Here's how the part is built. I have some questions about the finished solid (model axes, mm). A direction names the side the tool comes from. Round coordinates to 2 decimals unless told otherwise and drop trailing zeros. Loops run counter-clockwise (first coordinate to the right, second up) from the corner with the lowest first, then second, coordinate; pieces in that order, holes last. Notation, with made-up numbers: M 82,88.25 L 129,88.25 A25 ccw 129,101.25 Z; hole C 48.25,11 d11. An arc over 180 degrees is marked long. Put each result on its own line as item: value. Start each with the question number.
```python
from build123d import *

# Parameters (mm, degrees)
SKETCH_1_R          = 2
SKETCH_1_R_2        = 1
EXTRUDE_1_DEPTH     = 29
SKETCH_2_R          = 3
SKETCH_2_R_2        = 2
EXTRUDE_2_DEPTH     = 2.5
EXTRUDE_START       = 26.5
SKETCH_3_R          = 3
SKETCH_3_R_2        = 2
EXTRUDE_3_DEPTH     = 2.5
SKETCH_4_R          = 1.6
CUT_EXTRUDE_1_DEPTH = 1.5
CUT_EXTRUDE_START   = 29
CUT_EXTRUDE_2_DEPTH = 1.6
CUT_EXTRUDE_START_2 = 18.5
SKETCH_7_R          = 3
CUT_EXTRUDE_3_DEPTH = 10.5
CUT_EXTRUDE_START_3 = 10.5
CUT_EXTRUDE_5_DEPTH = 8


with BuildPart() as part:
    # 草图1 → 凸台-拉伸1 (new body)
    with BuildSketch(Plane(origin=(0, 0, 0), x_dir=(1, 0, 0), z_dir=(0, 1, 0))):
        with Locations(Location((0, 0, 0), (0, 0, 90))):
            Circle(SKETCH_1_R)
        with Locations(Location((0, 0, 0), (0, 0, 90))):
            Circle(SKETCH_1_R_2, mode=Mode.SUBTRACT)
    extrude(amount=EXTRUDE_1_DEPTH)

    # 草图2 → 凸台-拉伸2 (add)
    with BuildSketch(Plane(origin=(0, 0, 0), x_dir=(1, 0, 0), z_dir=(0, 1, 0))):
        with Locations(Location((0, 0, 0), (0, 0, 270))):
            Circle(SKETCH_2_R)
        with Locations(Location((0, 0, 0), (0, 0, 90))):
            Circle(SKETCH_2_R_2, mode=Mode.SUBTRACT)
    extrude(amount=EXTRUDE_2_DEPTH)

    # 草图3 → 凸台-拉伸3 (add)
    with BuildSketch(Plane(origin=(0, 0, 0), x_dir=(1, 0, 0), z_dir=(0, 1, 0)).offset(EXTRUDE_START)):
        with Locations(Location((0, 0, 0), (0, 0, 270))):
            Circle(SKETCH_3_R)
        with Locations(Location((0, 0, 0), (0, 0, 90))):
            Circle(SKETCH_3_R_2, mode=Mode.SUBTRACT)
    extrude(amount=EXTRUDE_3_DEPTH)

    # 草图4 → 切除-拉伸1 (cut)
    with BuildSketch(Plane(origin=(0, 0, 0), x_dir=(1, 0, 0), z_dir=(0, 1, 0))):
        with Locations(Location((0, 0, 0), (0, 0, 270))):
            Circle(SKETCH_4_R)
    extrude(amount=CUT_EXTRUDE_1_DEPTH, mode=Mode.SUBTRACT)

    # 草图5 → 切除-拉伸2 (cut)
    with BuildSketch(Plane(origin=(0, 0, 0), x_dir=(1, 0, 0), z_dir=(0, 1, 0)).offset(CUT_EXTRUDE_START)):
        Polygon((0, -2.309401077), (2, -1.154700538), (2, 1.154700538), (0, 2.309401077), (-2, 1.154700538), (-2, -1.154700538), align=None)
    extrude(amount=-CUT_EXTRUDE_2_DEPTH, mode=Mode.SUBTRACT)

    # 草图7 → 切除-拉伸3 (cut)
    with BuildSketch(Plane(origin=(0, 0, 0), x_dir=(1, 0, 0), z_dir=(0, 1, 0)).offset(CUT_EXTRUDE_START_2)):
        with Locations(Location((0, 0, 0), (0, 0, 270))):
            Circle(SKETCH_7_R)
    extrude(amount=CUT_EXTRUDE_3_DEPTH, mode=Mode.SUBTRACT)

    # 草图8 → 切除-拉伸5 (cut)
    with BuildSketch(Plane(origin=(0, 0, 0), x_dir=(1, 0, 0), z_dir=(0, 1, 0)).offset(CUT_EXTRUDE_START_3)):
        with BuildLine():
            ThreePointArc((0, -2), (1.414213562, -1.414213562), (2, 0))
            Line((2, 0), (0, 0))
            Line((0, 0), (0, -2))
        make_face()
        with BuildLine():
            Line((-2, 0), (0, 0))
            Line((0, 0), (0, 2))
            ThreePointArc((0, 2), (-1.414213562, 1.414213562), (-2, 0))
        make_face()
    extrude(amount=CUT_EXTRUDE_5_DEPTH, mode=Mode.SUBTRACT)


solid = part.part
```
1) Suppose I cut it at D-D (z = -2.35). Write out the boundary of the cut face in (x, y).
2) On a 3-axis mill with a long thin cutter (end or side, diameter ignored), from which of +Z, -Z, +X, -X, +Y, -Y can I reach the whole of each face in a straight line? I mean faces 1 (the face through (-1.5, 14.4, 0)), 2 (the face through (-1, 2.5, 2)), 3 (the face through (1, 10.5, 1)). Say none if no direction works.
3) I'm going to push flat-ended pins straight in: P1, Ø0.8, axis at y = 13.5, z = 1.5, coming from the +X side; P2, Ø0.5, axis at y = 13, z = -1.5, coming from the -X side; P3, Ø0.8, axis at x = -1.5, y = 13.5, coming from the -Z side; P4, Ø1.6, axis at x = 0, z = 0, coming from the -Y side. Where does each tip first touch, or does it pass through?
4) Suppose I cut it at C-C (x = 2.4). Write out the boundary of the cut face in (y, z), plus the area to 3 significant figures.
5) If I drill on probe 1 along X at (y, z) = (6.5, 0); probe 2 along X at (y, z) = (0.45, 0); probe 3 along Y at (x, z) = (-2.25, -1.55), over which ranges is the centre line in solid material (lowest first)? Write a range as from..to.
6) Suppose I cut it at A-A (z = -0.3). Write out the boundary of the cut face in (x, y), plus the area to 3 significant figures.
7) If we mould it in two halves opening along X, with no side actions, what happens to faces 4 (the face through (-0.97, 0.74, -1.27)), 5 (the face through (1.5, 14.4, 0)), 6 (the face through (0.9, 1.23, 2.86))? For each: pulls with the +X half, pulls with the -X half, needs draft (parallel to the pull), parting line crosses it, or undercut.
8) Suppose I cut it at B-B (y = 9.75). Write out the boundary of the cut face in (x, z).
Results are:
1. outline: M -1.86,0 L 1.86,0 L 1.86,2.5 L -1.86,2.5 Z
2. face 1: -Z, -X, +Y
2. face 2: +Y
2. face 3: +Z, +X, +Y
3. P1: x = 0
3. P2: x = 0
3. P3: z = 0
3. P4: through
4. outline: M 0,-1.8 L 2.5,-1.8 L 2.5,1.8 L 0,1.8 Z
4. area: 9.00 mm²
5. probe 1: -2..-1, 1..2
5. probe 2: -3..-1.6, 1.6..3
5. probe 3: 0..2.5
6. outline: M -2.98,0 L -1.57,0 L -1.57,1.5 L -0.95,1.5 L -0.95,10.5 L -1.98,10.5 L -1.98,2.5 L -2.98,2.5 Z; M 0.95,1.5 L 1.57,1.5 L 1.57,0 L 2.98,0 L 2.98,2.5 L 1.98,2.5 L 1.98,18.5 L 0.95,18.5 Z
6. area: 32.9 mm²
7. face 4: undercut
7. face 5: needs draft
7. face 6: parting line crosses it
8. outline: C 0,0 d4; hole C 0,0 d2
